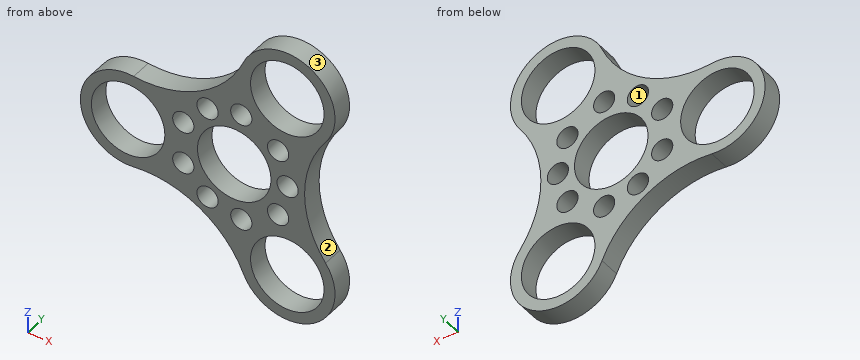
from build123d import *

# Parameters (mm, degrees)
F2_R     = 10.9982
F2_R_2   = 14.2875
F3_DEPTH = 6.35
F4_R     = 3.175
F5_R     = 3.175
F6_DEPTH = 6.351


with BuildPart() as f3:
    # F2 (on Front) → F3 (new body)
    with BuildSketch(Plane.XZ):
        with BuildLine():
            ThreePointArc((30.1625, 27.4963065702), (18.7633086309, 41.4888163344), (2.7552797722, 33.1536555423))
            ThreePointArc((2.7552797722, 33.1536555423), (8.73125, 15.1229686136), (27.3342680419, 18.9629700484))
            ThreePointArc((27.3342680419, 18.9629700484), (29.437023234, 23.0014003364), (30.1625, 27.4963065702))
        make_face()
        with Locations((15.875, 27.4963065702)):
            Circle(F2_R, mode=Mode.SUBTRACT)
        with BuildLine():
            ThreePointArc((-30.0895478141, 14.1906854939), (-21.0762853969, 9.4976035305), (-17.4625, 0))
            ThreePointArc((-17.4625, 0), (-21.0762853969, -9.4976035305), (-30.0895478141, -14.1906854939))
            ThreePointArc((-30.0895478141, -14.1906854939), (-10.5246540675, -18.229235577), (2.7552797722, -33.1536555423))
            ThreePointArc((2.7552797722, -33.1536555423), (8.73125, -15.1229686136), (27.3342680419, -18.9629700484))
            ThreePointArc((27.3342680419, -18.9629700484), (21.049308135, 0), (27.3342680419, 18.9629700484))
            ThreePointArc((27.3342680419, 18.9629700484), (8.73125, 15.1229686136), (2.7552797722, 33.1536555423))
            ThreePointArc((2.7552797722, 33.1536555423), (-10.5246540675, 18.229235577), (-30.0895478141, 14.1906854939))
        make_face()
        Circle(F2_R_2, mode=Mode.SUBTRACT)
        Circle(F2_R_2)
        Circle(F2_R, mode=Mode.SUBTRACT)
        with BuildLine():
            ThreePointArc((-30.0895478141, -14.1906854939), (-21.0762853969, -9.4976035305), (-17.4625, 0))
            ThreePointArc((-17.4625, 0), (-21.0762853969, 9.4976035305), (-30.0895478141, 14.1906854939))
            ThreePointArc((-30.0895478141, 14.1906854939), (-46.0375, 0), (-30.0895478141, -14.1906854939))
        make_face()
        with Locations((-31.75, 0)):
            Circle(F2_R, mode=Mode.SUBTRACT)
        with BuildLine():
            ThreePointArc((27.3342680419, -18.9629700484), (8.73125, -15.1229686136), (2.7552797722, -33.1536555423))
            ThreePointArc((2.7552797722, -33.1536555423), (18.7633086309, -41.4888163344), (30.1625, -27.4963065702))
            ThreePointArc((30.1625, -27.4963065702), (29.437023234, -23.0014003364), (27.3342680419, -18.9629700484))
        make_face()
        with Locations((15.875, -27.4963065702)):
            Circle(F2_R, mode=Mode.SUBTRACT)
    extrude(amount=F3_DEPTH)

    # F4 (on face) + F5 (on face) → F6 (cut, through all)
    with BuildSketch(Plane.XZ.offset(6.35)):
        with Locations((-15.24, 6.35)):
            Circle(F4_R)
        with Locations((2.120738686, 16.3732271537)):
            Circle(F4_R)
        with Locations((13.119261314, 10.0232271537)):
            Circle(F4_R)
        with Locations((13.119261314, -10.0232271537)):
            Circle(F4_R)
        with Locations((2.120738686, -16.3732271537)):
            Circle(F4_R)
        with Locations((-15.24, -6.35)):
            Circle(F4_R)
    with BuildSketch(Plane.XZ.offset(6.35)):
        with Locations((-7.9846540675, 13.8298265258)):
            Circle(F5_R)
        with Locations((15.969308135, 0)):
            Circle(F5_R)
        with Locations((-7.9846540675, -13.8298265258)):
            Circle(F5_R)
    extrude(amount=-F6_DEPTH, mode=Mode.SUBTRACT)


solid = f3.part
Could you check a few things on this model? Use its own coordinates, in mm. Face numbers are marked on the shaded views. Give positions to 0.01 mm unless a question says otherwise; leave off trailing zeros. Order: outer loops, then holes, each group sorted by start corner. A loop starts at its lowest first (then second) coordinate and runs counter-clockwise, first axis right, second up.
Item 1: If we section it at D-D, the plane z = 21.5: Write out the boundary of the cut face in (x, y).
Item 2: If we section it at C-C, the plane x = -15.24: Write out the boundary of the cut face in (y, z) (3 decimals), plus the area to 3 significant figures.
Item 3: I'm going to push flat-ended pins straight in: pin 1 (20 mm diameter, centred on x = 0, z = 0, fed in from +Y); pin 2 (1 mm diameter, centred on x = -10.5, y = -3, fed in from -Z); pin 3 (3 mm diameter, centred on y = -4, z = 2.5, fed in from +X); pin 4 (1.5 mm diameter, centred on x = -29, y = -1, fed in from +Z). Where does each tip first touch, or does it pass through?
Item 4: I need wall thicknesses on line 1 (Z direction, x = 25.5, y = -1.5); line 2 (Z direction, x = -31.75, y = -1.25); line 3 (Z direction, x = -6, y = -4). Which ranges of each line are inside material? Lowest first, please.
Item 5: If we section it at A-A, the plane x = -31.75: Write out the boundary of the cut face in (y, z), plus the area to 3 significant figures.
Item 6: If we section it at B-B, the plane z = 0: Write out the boundary of the cut face in (x, y), plus the area to 3 significant figures.
Item 7: If we mould it in two halves opening along X, with no side actions, what happens to the marked faces 1, 2 and 3? For each: pulls with the +X half, pulls with the -X half, needs draft (parallel to the pull), parting line crosses it, or undercut.
Values:
1. outline: (-5.88, -6.35) - (6.66, -6.35) - (6.66, 0) - (-5.88, 0) - close; (25.09, -6.35) - (28.84, -6.35) - (28.84, 0) - (25.09, 0) - close
2. outline: (-6.35, -16.001) - (0, -16.001) - (0, -9.525) - (-6.35, -9.525) - close; (-6.35, -3.175) - (0, -3.175) - (0, 3.175) - (-6.35, 3.175) - close; (-6.35, 9.525) - (0, 9.525) - (0, 16.001) - (-6.35, 16.001) - close
2. area: 123 mm2
3. pin 1: passes through
3. pin 2: stops at z = -18.54
3. pin 3: stops at x = 21.3
3. pin 4: stops at z = 14.15
4. line 1: z = -38.06 to -32.82, -22.17 to -16.21, 16.21 to 22.17, 32.82 to 38.06
4. line 2: z = -14.29 to -11, 11 to 14.29
4. line 3: z = -21.4 to -16.31, -11.35 to -9.22, 9.22 to 11.35, 16.31 to 21.4
5. outline: (-6.35, -14.29) - (0, -14.29) - (0, -11) - (-6.35, -11) - close; (-6.35, 11) - (0, 11) - (0, 14.29) - (-6.35, 14.29) - close
5. area: 41.8 mm2
6. outline: (-46.04, -6.35) - (-42.75, -6.35) - (-42.75, 0) - (-46.04, 0) - close; (-20.75, -6.35) - (-11, -6.35) - (-11, 0) - (-20.75, 0) - close; (11, -6.35) - (12.79, -6.35) - (12.79, 0) - (11, 0) - close; (19.14, -6.35) - (21.05, -6.35) - (21.05, 0) - (19.14, 0) - close
6. area: 106 mm2
7. face 1: undercut
7. face 2: pulls with the +X half
7. face 3: parting line crosses it
